Verification items for this drawing (mm, ordinates from the low corner). A direction names the side the tool comes from. Coordinates: 2 decimals unless noted, no trailing zeros. Write each loop counter-clockwise with the first axis right and the second up, starting at its lowest first coordinate (ties: lowest second). Pieces come first, ordered by that corner, then holes. Notation, with made-up numbers: (-33.5, 86) -> (-25.5, 86) arc R22 cw to (-25.5, 112) -> close; hole circle Ø4 at (-29.5, 19). An arc over 180 degrees is marked (long way). One line per item, written item: value. Start each with the question number.
1) Sectioned sample at D-D on x = 88. Enter the section's corners in (y, z).
2) Sectioned sample at B-B on z = 10.7. Enter the section's corners in (x, y).
3) Sectioned sample at A-A on y = 15. Enter the section's corners in (x, z).
4) Gauge pin test, flat ends, axial feed: P1, Ø1.2, axis at x = 4.5, z = 18, coming from the +Y side; P2, Ø8.5, axis at y = 17, z = 11, coming from the -X side; P3, Ø1.2, axis at y = 63.5, z = 19.5, coming from the +X side. Record the tip position at first contact, or that the pin passes through.
5) Set-up check for the marked faces 1 and 2: record each of +Z, -Z, +X, -X, +Y, -Y from which the full face is reachable in a straight line by a thin tool's end or side.
6) Sectioned sample at C-C on x = 21. Enter the section's corners in (y, z).
7) Scan lines: line 1 along Y through (x, z) = (21, 18.3); line 2 along X through (y, z) = (29.5, 17.5); line 3 along X through (y, z) = (24, 16). Record each from-to range of solid material in increasing order. Write a range as [from, to].
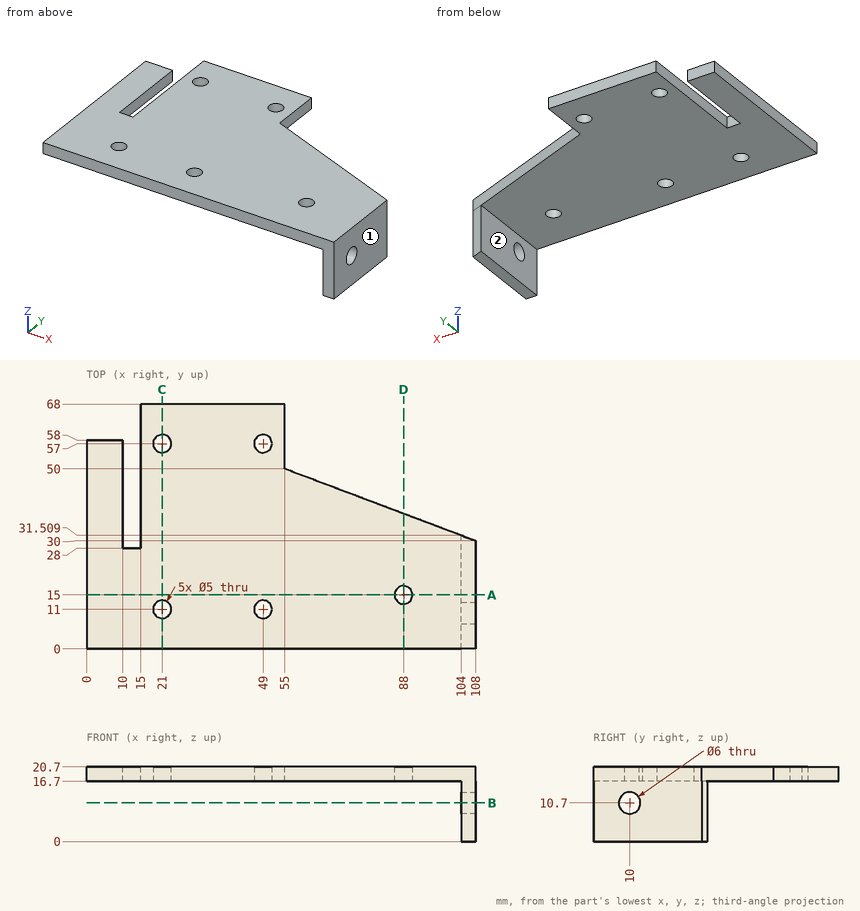
Answers:
1. outline: (0, 16.7) -> (12.5, 16.7) -> (12.5, 20.7) -> (0, 20.7) -> close; (17.5, 16.7) -> (37.55, 16.7) -> (37.55, 20.7) -> (17.5, 20.7) -> close
2. outline: (104, 0) -> (108, 0) -> (108, 7) -> (104, 7) -> close; (104, 13) -> (108, 13) -> (108, 30) -> (104, 31.51) -> close
3. outline: (0, 16.7) -> (85.5, 16.7) -> (85.5, 20.7) -> (0, 20.7) -> close; (90.5, 16.7) -> (104, 16.7) -> (104, 0) -> (108, 0) -> (108, 20.7) -> (90.5, 20.7) -> close
4. P1: stops at y = 58
4. P2: stops at x = 104
4. P3: stops at x = 55
5. face 1: +Z, -Z, +X, +Y, -Y
5. face 2: -Z, -X, +Y, -Y
6. outline: (0, 16.7) -> (8.5, 16.7) -> (8.5, 20.7) -> (0, 20.7) -> close; (13.5, 16.7) -> (54.5, 16.7) -> (54.5, 20.7) -> (13.5, 20.7) -> close; (59.5, 16.7) -> (68, 16.7) -> (68, 20.7) -> (59.5, 20.7) -> close
7. line 1: y = [0, 8.5], [13.5, 54.5], [59.5, 68]
7. line 2: x = [0, 10], [15, 108]
7. line 3: x = [104, 108]
